Can you work these out from the model? Positions are in its coordinate system, mm. Give positions to 0.01 mm unless a question says otherwise; leave off trailing zeros. Loops run counter-clockwise (first coordinate to the right, second up) from the corner with the lowest first, then second, coordinate; pieces in that order, holes last. Notation, with made-up numbers: (-14.5, -5.75) -> (-7.5, -5.75) arc R11 ccw to (-7.5, 6.25) -> close; hole circle Ø9 at (12.5, 1.5). An arc over 180 degrees is marked (long way). Use CSV: the item, a comma, the result in double quotes.
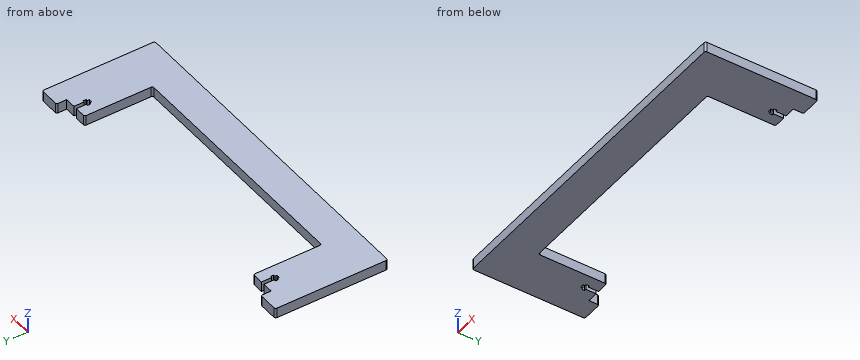
Autodesk Inventor part; units mm, degrees
ref_plane "YZ Plane" through (0, 0, 0) normal (1, 0, 0) x (0, 1, 0)
ref_plane "XZ Plane" through (0, 0, 0) normal (0, 1, 0) x (-1, 0, 0)
ref_plane "XY Plane" through (0, 0, 0) normal (0, 0, 1) x (1, 0, 0)
sketch "Sketch1" plane through (0, 0, 0) normal (0, 0, 1) x (1, 0, 0)
  line L0 (100, -30) -> (-100, -30)
  line L1 (-100, -30) -> (-100, 30)
  line L2 (-100, 30) -> (100, 30)
  line L3 (100, 30) -> (100, -30)
  line L4 (100, -30) -> (-100, 30) construction
  line L5 (-100, -30) -> (100, 30) construction
  point P0 (0, 0)
  dimension "d0" = 200
  dimension "d1" = 60
extrude "Extrusion1" add sketch "Sketch1" along normal blind 6
sketch "Sketch2" plane through (0, 0, 6) normal (0, 0, 1) x (1, 0, 0)
  line L0 (-100, -30) -> (100, -30)
  line L1 (100, 30) -> (-100, 30)
  line L2 (-72.5, -10) -> (72.5, -10)
  line L3 (72.5, -10) -> (72.5, 30)
  line L4 (72.5, 30) -> (-72.5, 30)
  line L5 (-72.5, 30) -> (-72.5, -10)
  line L6 (-72.5, -10) -> (72.5, 30) construction
  line L7 (72.5, -10) -> (-72.5, 30) construction
  point P0 (0, 0)
  point P1 (0, 10)
  dimension "d4" = 145
  dimension "d5" = 20
extrude "Extrusion2" cut sketch "Sketch2" against normal through all
sketch "Sketch3" plane through (0, 0, 6) normal (0, 0, 1) x (1, 0, 0)
  line L0 (100, 30) -> (72.5, 30)
  line L1 (-100, 30) -> (-87.75, 30)
  line L2 (-87.75, 30) -> (-87.75, 36)
  line L3 (-87.75, 36) -> (-100, 36)
  line L4 (-100, 36) -> (-100, 30)
  line L5 (100, 30) -> (87.75, 30)
  line L6 (87.75, 30) -> (87.75, 36)
  line L7 (87.75, 36) -> (100, 36)
  line L8 (100, 36) -> (100, 30)
  point P0 (0, 0)
  dimension "d9" = 6
  dimension "d20" = 12.25
extrude "Extrusion3" add sketch "Sketch3" against normal up to surface (6 mm away)
sketch "Sketch4" plane through (0, 0, 6) normal (0, 0, 1) x (1, 0, 0)
  line L0 (-72.5, 30) -> (-87.75, 30)
  line L1 (-81.55, 30) -> (-81.55, 24)
  line L2 (-81.55, 24) -> (-82.55, 24)
  line L3 (-82.55, 24) -> (-82.55, 22.2)
  line L4 (-82.55, 22.2) -> (-81.55, 22.2)
  line L5 (-81.55, 22.2) -> (-81.55, 21)
  line L6 (-81.55, 21) -> (-79.45, 21)
  line L7 (-79.45, 21) -> (-79.45, 22.2)
  line L8 (-79.45, 22.2) -> (-78.45, 22.2)
  line L9 (-78.45, 22.2) -> (-78.45, 24)
  line L10 (-78.45, 24) -> (-79.45, 24)
  line L11 (-79.45, 24) -> (-79.45, 30)
  line L12 (-72.5, -10) -> (-72.5, 30)
  line L13 (72.5, -10) -> (-72.5, -10)
  line L14 (-80.5, 21) -> (-80.5, 27.2544) construction
  line L15 (-79.45, 30) -> (-81.55, 30)
  point P0 (0, 0)
  point P1 (-80.125, 30)
  dimension "d12" = 2.1
  dimension "d13" = 4.1
  dimension "d15" = 6
  dimension "d16" = 1.8
  dimension "d21" = 8
  dimension "d22" = 9
extrude "Extrusion4" cut sketch "Sketch4" against normal blind 10
mirror "Mirror1" about plane through (0, 0, 0) normal (1, 0, 0) of "Extrusion4"
fillet "Fillet1" radius 1 10 edges at (-100, 36, 3) (-87.75, 36, 3) (-72.5, 30, 3) (72.5, 30, 3) (87.75, 36, 3) (100, 36, 3) (100, -30, 3) (72.5, -10, 3) (-72.5, -10, 3) (-100, -30, 3)
properties part number "InnerFront"
(1) If I drill on L1, parallel to X at y = 21.5, z = 5.6; L2, parallel to Y at x = 32, z = 3.45; L3, parallel to X at y = 8, z = 1.3, over which ranges is the centre line in solid material (lowest first)? Write a range as from..to.
Answer sheet:
L1,"x = -100..-81.55, -79.45..-72.5, 72.5..79.45, 81.55..100"
L2,"y = -30..-10"
L3,"x = -100..-72.5, 72.5..100"
(2) If we section it at A-A, the plane y = 18: Write out the boundary of the cut face in (x, z), then the cut area to 3 significant figures.
Answer sheet:
outline,"(-100, 0) -> (-72.5, 0) -> (-72.5, 6) -> (-100, 6) -> close; (72.5, 0) -> (100, 0) -> (100, 6) -> (72.5, 6) -> close"
area,"330 mm2"
(3) If we section it at B-B, the plane x = -30: Write out the boundary of the cut face in (y, z), then the cut area to 3 significant figures.
Answer sheet:
outline,"(-30, 0) -> (-10, 0) -> (-10, 6) -> (-30, 6) -> close"
area,"120 mm2"
(4) Will this pin go through, and if not, where does the flat tip stop? pin 1 Ø0.5 at (x, z) = (79, 3) entering from +Y.
Answer sheet:
pin 1,"stops at y = 30"
